CAD build for the part. Positions are in the model's coordinates, mm. Face numbers are marked on the shaded views. A direction names the side the tool comes from. Round coordinates to 2 decimals unless told otherwise and drop trailing zeros. Loops run counter-clockwise (first coordinate to the right, second up) from the corner with the lowest first, then second, coordinate; pieces in that order, holes last. Notation, with made-up numbers: M 47,68.5 L 80,68.5 A20 ccw 80,80.5 Z; hole C 55,66 d1. An arc over 180 degrees is marked long. Use one line per item in the form item = value.
from build123d import *

# Parameters (mm, degrees)
BASPROSKE_W             = 7
BASPROSKE_H             = 7.7
TOOTHCUT_DEPTH          = 13.945269406
TEETHCUTS_COUNT         = 20
TEETHCUTS_ANGLE         = 342
BORSKE_R                = 0.5
BORE_DEPTH              = 50.0000508
CUT_EXTRUDE1_DEPTH      = 13.86365753
CUT_EXTRUDE1_DEPTH_BACK = 13.86365753
SKETCH1_W               = 3.8
SKETCH1_H               = 5.3


with BuildPart() as part:
    # BasProSke → Base-Revolve (revolve)
    with BuildSketch(Plane(origin=(0, 0, 0), x_dir=(1, 0, 0), z_dir=(0, 1, 0)), mode=Mode.PRIVATE) as base_revolve_sk:
        with Locations((3.5, 3.85)):
            Rectangle(BASPROSKE_W, BASPROSKE_H)
    revolve(base_revolve_sk.sketch.rotate(Axis((-10, 0, 0), (1, 0, 0)), 180), axis=Axis((-10, 0, 0), (1, 0, 0)))

    # TooCutSke → ToothCut (cut, through all)
    with BuildSketch(Plane(origin=(0, 0, 0), x_dir=(0, 0, -1), z_dir=(1, 0, 0))):
        with BuildLine():
            ThreePointArc((0.350524468, 6.11396014), (0, 6.124), (-0.350524468, 6.11396014))
            ThreePointArc((-0.350524468, 6.11396014), (-0.579534642, 6.937844235), (-1.04652851, 7.654187301))
            ThreePointArc((-1.04652851, 7.654187301), (0, 7.7254), (1.04652851, 7.654187301))
            ThreePointArc((1.04652851, 7.654187301), (0.579534642, 6.937844235), (0.350524468, 6.11396014))
        make_face()
    toothcut = extrude(amount=TOOTHCUT_DEPTH, mode=Mode.SUBTRACT)

    # TeethCuts: ToothCut ×20 about axis
    teethcuts_axis = Axis((-10, 0, 0), (1, 0, 0))
    for i in range(1, TEETHCUTS_COUNT):
        add(toothcut.rotate(teethcuts_axis, i * TEETHCUTS_ANGLE / (TEETHCUTS_COUNT - 1)), mode=Mode.SUBTRACT)

    # BorSke → Bore (cut, symmetric)
    with BuildSketch(Plane(origin=(0, 0, 0), x_dir=(0, 0, -1), z_dir=(1, 0, 0))):
        with Locations(Location((0, 0, 0), (0, 0, 180))):
            Circle(BORSKE_R)
    extrude(amount=BORE_DEPTH, both=True, mode=Mode.SUBTRACT)

    # Sketch1 → Cut-Extrude1 (cut, two sides: drawn at the far end of the back side and taken through both)
    with BuildSketch(Plane(origin=(7, 0, 0), x_dir=(0, 0, -1), z_dir=(1, 0, 0)).offset(-CUT_EXTRUDE1_DEPTH_BACK)):
        Rectangle(SKETCH1_W, SKETCH1_H)
    extrude(amount=CUT_EXTRUDE1_DEPTH + CUT_EXTRUDE1_DEPTH_BACK, mode=Mode.SUBTRACT)


solid = part.part
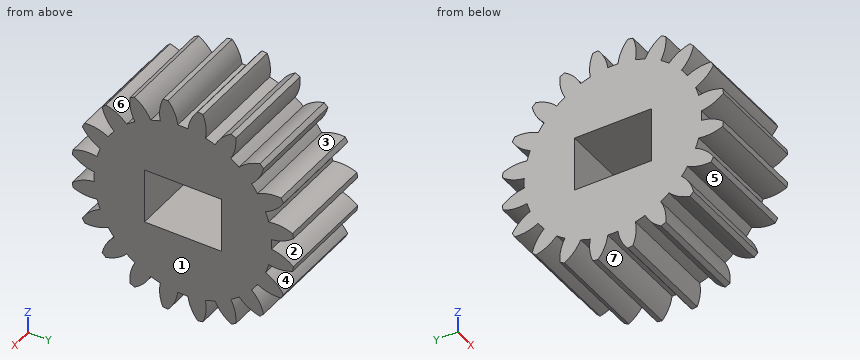
1. Tool access for the marked faces 4, 5, 6 and 7: list every direction of +Z, -Z, +X, -X, +Y, -Y with a clear straight run to the whole face (end or side of a thin tool).
Completed:
face_4 = +X, -X, +Y
face_5 = +X, -X
face_6 = +Z, +X, -X
face_7 = -Z, +X, -X
2. Cut at C-C on y = 3. Write the cut outline in (x, z).
Completed:
outline = M 0,-6.71 L 7,-6.71 L 7,6.71 L 0,6.71 Z
3. Probe line 1 along Z through (x, y) = (2.75, 0); line 2 along Z through (x, y) = (6, -6.75); line 3 along Z through (x, y) = (3.5, -6.25). List the from-to ranges inside material, lowest first. Write a range as from..to.
Completed:
line_1 = -6.12..-1.9, 1.9..6.12
line_2 = -3.66..-3.05, -1.6..-0.5, 0.5..1.6, 3.05..3.66
line_3 = -3.65..-2.55, -1.6..-0.37, 0.37..1.6, 2.55..3.65
4. Cut at B-B on z = -6.5. Write the cut outline in (x, y).
Completed:
outline = M 0,-3.67 L 7,-3.67 L 7,-2.77 L 0,-2.77 Z; M 0,-1.61 L 7,-1.61 L 7,-0.42 L 0,-0.42 Z; M 0,0.42 L 7,0.42 L 7,1.61 L 0,1.61 Z; M 0,2.77 L 7,2.77 L 7,3.67 L 0,3.67 Z
5. Drop flat-ended pins along their axis: P1, Ø2.5, axis at x = 3, y = 0, coming from the +Z side; P2, Ø3, axis at x = 5, z = -6, coming from the -Y side. Give the stop position or say it passes through.
Completed:
P1 = 7.63
P2 = -5.57
6. Pull direction Y, two halves, no side cores. Call the marked faces 1, 2 and 3: +Y half, -Y half, draft (parallel to the pull), parting line (faces both ways), or undercut.
Completed:
face_1 = draft
face_2 = +Y half
face_3 = undercut
7. Cut at A-A on z = 0. Write the cut outline in (x, y), and give its area (3 significant figures).
Completed:
outline = M 0,-6.12 L 7,-6.12 L 7,-2.65 L 0,-2.65 Z; M 0,2.65 L 7,2.65 L 7,6.12 L 0,6.12 Z
area = 48.6 mm2
